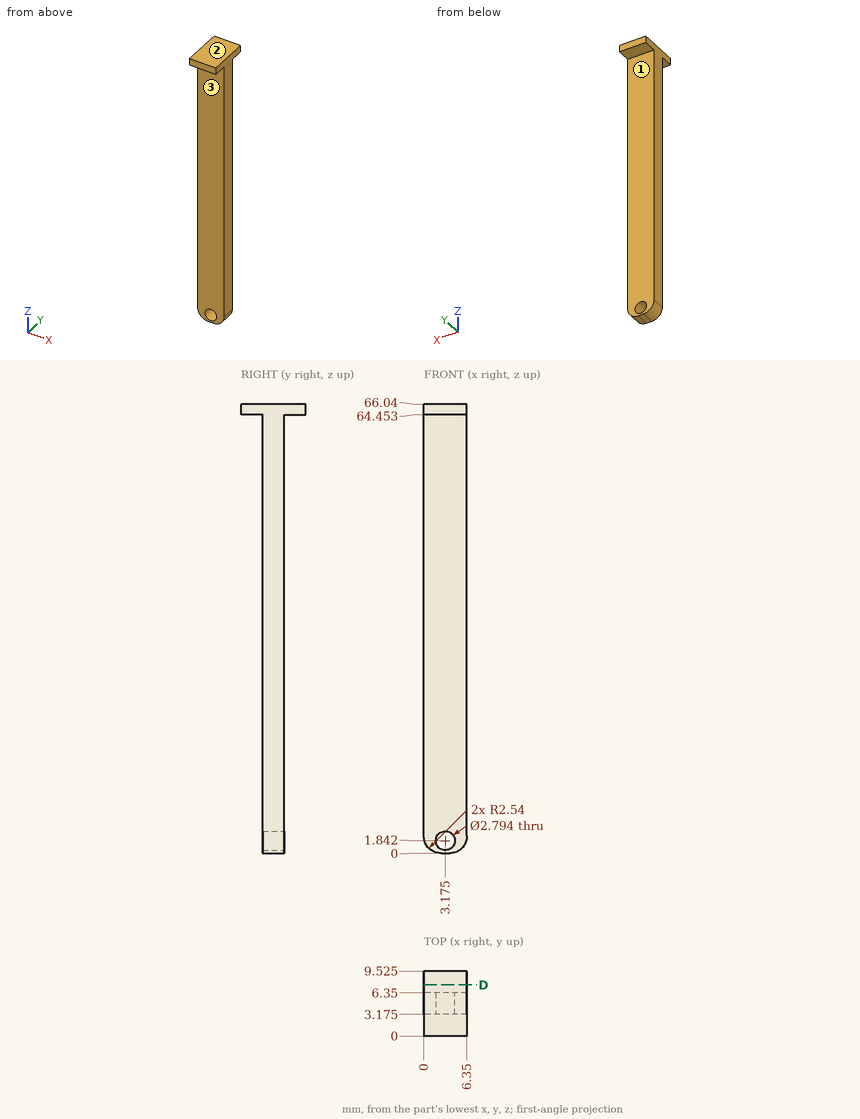
Verification items for this drawing (mm, ordinates from the low corner). A direction names the side the tool comes from. Coordinates: 2 decimals unless noted, no trailing zeros. Loops run counter-clockwise (first coordinate to the right, second up) from the corner with the lowest first, then second, coordinate; pieces in that order, holes last. Notation, with made-up numbers: (89, 74) - (147, 74) arc R35 ccw to (147, 111) - close; hole circle Ø2 at (42, 20.5). An arc over 180 degrees is marked (long way). One line per item, written item: value. Start each with the question number.
(1) Cross-section at D-D on y = 7.5. Enter the section's corners in (x, z), plus the area to 3 significant figures.
(2) Material ranges on line 1 (Z direction, x = 4.5, y = 6.5); line 2 (Z direction, x = 1.5, y = 6), recorded low to high. Write a range as [from, to].
(3) Depth check by flat-ended pin: P1, Ø2.5, axis at x = 3.5, y = 8, coming from the -Z side; P2, Ø2, axis at x = 4, z = 37.5, coming from the +Y side; P3, Ø2.5, axis at x = 3.18, z = 1.84, coming from the -Y side. Enter the tip coordinate at first touch or a pass-through.
(4) Tool access check on the marked faces 1, 2 and 3. Record the directions out of +Z, -Z, +X, -X, +Y, -Y that give a thin tool (end or side, any length) a straight path to the whole face; none if there is none.
Results below:
1. outline: (0, 64.45) - (6.35, 64.45) - (6.35, 66.04) - (0, 66.04) - close
1. area: 10.1 mm2
2. line 1: z = [64.45, 66.04]
2. line 2: z = [0.22, 66.04]
3. P1: stops at z = 64.45
3. P2: stops at y = 6.35
3. P3: passes through
4. face 1: -Z, +X, -X, +Y
4. face 2: +Z, +X, -X, +Y, -Y
4. face 3: -Z, +X, -X, -Y
